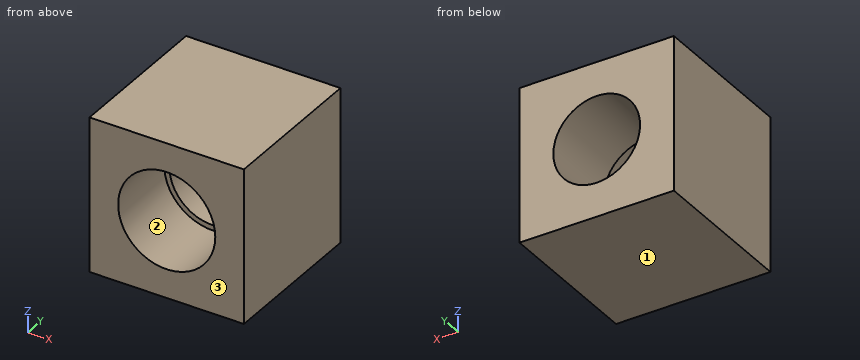
from build123d import *

# Parameters (mm, degrees)
SKETCH1_W           = 11.303
SKETCH1_H           = 11.303
SKETCH1_R           = 3.175
BOSS_EXTRUDE1_DEPTH = 11.176
CUT_EXTRUDE1_REACH  = 19.018
CUT_EXTRUDE1_START  = -5.842
SKETCH2_R           = 3.556
SKETCH2_R_2         = 3.175


with BuildPart() as part:
    # Sketch1 → Boss-Extrude1 (new body)
    with BuildSketch(Plane(origin=(0, 0, 0), x_dir=(1, 0, 0), z_dir=(0, 1, 0))):
        with Locations((5.6515, 5.6515)):
            Rectangle(SKETCH1_W, SKETCH1_H)
        with Locations((5.6515, 5.6515)):
            Circle(SKETCH1_R, mode=Mode.SUBTRACT)
    extrude(amount=BOSS_EXTRUDE1_DEPTH)

    # Sketch2 → Cut-Extrude1 (cut, up to next)
    with BuildSketch(Plane(origin=(0, 11.176, 0), x_dir=(1, 0, 0), z_dir=(0, 1, 0)).offset(CUT_EXTRUDE1_START), mode=Mode.PRIVATE) as cut_extrude1_sk1:
        with Locations((5.6515, 5.6515)):
            Circle(SKETCH2_R)
        with Locations((5.6515, 5.6515)):
            Circle(SKETCH2_R_2, mode=Mode.SUBTRACT)
    cut_extrude1_tool1 = extrude(cut_extrude1_sk1.sketch, amount=-CUT_EXTRUDE1_REACH, mode=Mode.PRIVATE) & part.part
    add(cut_extrude1_tool1.solids().sort_by_distance((2.196079, 5.334, -5.6515))[0], mode=Mode.SUBTRACT)


solid = part.part
Could you check a few things on this model? Use its own coordinates, in mm. Face numbers are marked on the shaded views. Give positions to 0.01 mm unless a question says otherwise; leave off trailing zeros. Order: outer loops, then holes, each group sorted by start corner. A loop starts at its lowest first (then second) coordinate and runs counter-clockwise, first axis right, second up.
Item 1: If we section it at A-A, the plane x = 6.75: Write out the boundary of the cut face in (y, z), plus the area to 3 significant figures.
Item 2: If we mould it in two halves opening along Z, with no side actions, what happens to the marked faces 1, 2 and 3? For each: pulls with the +Z half, pulls with the -Z half, needs draft (parallel to the pull), parting line crosses it, or undercut.
Item 3: If we section it at C-C, the plane y = 4.25: Write out the boundary of the cut face in (x, z), plus the area to 3 significant figures.
Item 4: I need wall thicknesses on line 1 (X direction, y = 6, z = -3.75); line 2 (Z direction, x = 7.75, y = 3.25); line 3 (X direction, y = 3.25, z = -3.5). Which ranges of each line are inside material? Lowest first, please.
Item 5: If we section it at B-B, the plane z = -8.5: Write out the boundary of the cut face in (x, y), plus the area to 3 significant figures.
Item 6: I'm going to push a flat-ended pin straight in: pin 1 (2 mm diameter, centred on x = 5, z = -6, fed in from -Y). Where does the tip first touch, or does it pass through?
Values:
1. outline: (0, -11.3) - (11.18, -11.3) - (11.18, -8.63) - (5.33, -8.63) - (5.33, -9.03) - (0, -9.03) - close; (0, -2.27) - (5.33, -2.27) - (5.33, -2.67) - (11.18, -2.67) - (11.18, 0) - (0, 0) - close
1. area: 55.4 mm2
2. face 1: pulls with the -Z half
2. face 2: undercut
2. face 3: needs draft
3. outline: (0, -11.3) - (11.3, -11.3) - (11.3, 0) - (0, 0) - close; hole circle Ø7.11 at (5.65, -5.65)
3. area: 88.0 mm2
4. line 1: x = 0 to 3.11, 8.19 to 11.3
4. line 2: z = -11.3 to -8.52, -2.78 to 0
4. line 3: x = 0 to 2.82, 8.48 to 11.3
5. outline: (0, 0) - (3.52, 0) - (3.52, 5.33) - (4.25, 5.33) - (4.25, 11.18) - (0, 11.18) - close; (7.05, 5.33) - (7.78, 5.33) - (7.78, 0) - (11.3, 0) - (11.3, 11.18) - (7.05, 11.18) - close
5. area: 87.2 mm2
6. pin 1: passes through
